Could you check a few things on this drawing? It's one solid part, dimensions in mm from its lowest x, y, z. A direction names the side the tool comes from. Coordinates: 2 decimals unless noted, no trailing zeros. Order: outer loops, then holes, each group sorted by start corner. A loop starts at its lowest first (then second) coordinate and runs counter-clockwise, first axis right, second up.
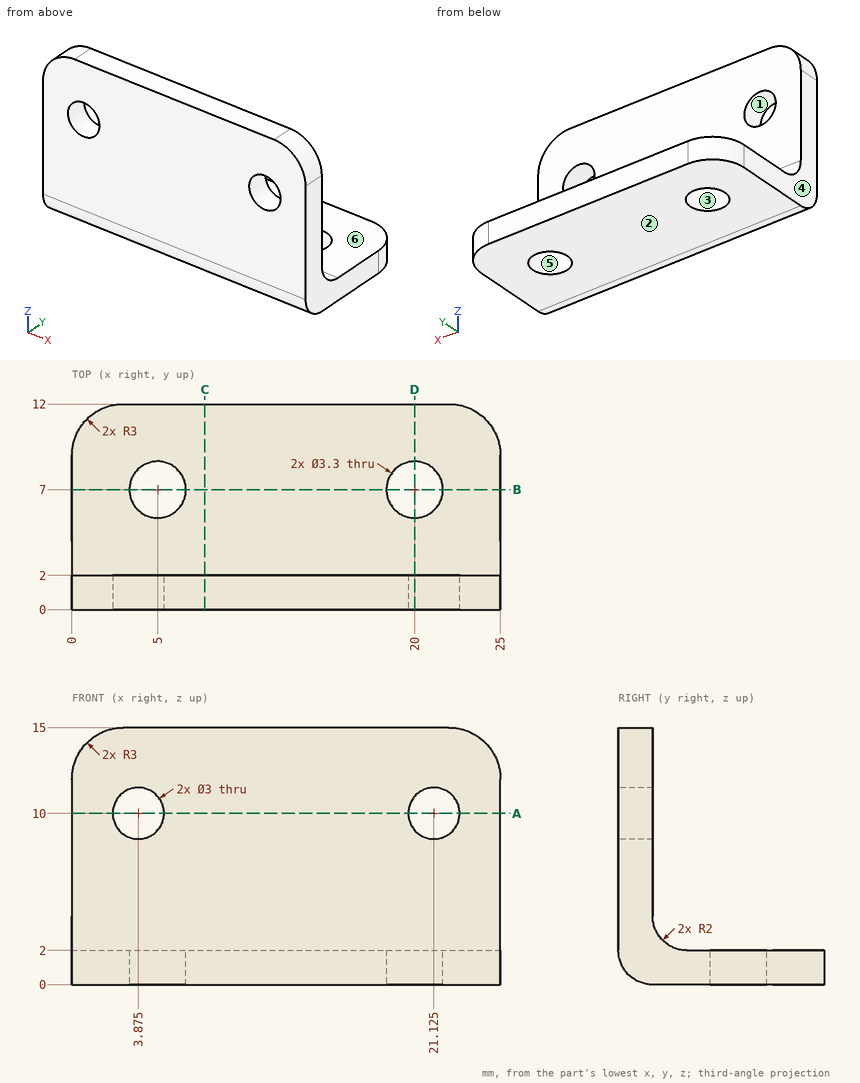
Item 1: Which directions (+Z, -Z, +X, -X, +Y, -Y) give clear straight access to the entire face, cutting with the end or side of a thin tool? Please do the marked faces 5 and 6.
Item 2: Suppose I cut it at D-D (x = 20). List the corners of the cut face in (y, z) for me.
Item 3: Suppose I cut it at C-C (x = 7.75). List the corners of the cut face in (y, z) for me.
Item 4: I need wall thicknesses on line 1 (X direction, y = 7, z = 1.35); line 2 (Y direction, x = 7.5, z = 9.75); line 3 (X direction, y = 1.75, z = 9.75). Which ranges of each line are inside material? Lowest first, please.
Item 5: For pin 1 Ø4 at (x, y) = (11.5, 8.5) entering from +Z; pin 2 Ø9 at (x, z) = (6.5, 7.5) entering from +Y, each with a flat end and sliding along its axis, tell me the tip position at first contact or that it passes through.
Item 6: Thinking about a two-plate mould opening in X: for the marked faces 1, 2, 3 and 4, which applies, +X half, -X half, draft (parallel to the pull), parting line (faces both ways), or undercut?
Item 7: Suppose I cut it at B-B (y = 7). List the corners of the cut face in (x, z) for me.
Item 8: Suppose I cut it at A-A (z = 10). List the corners of the cut face in (x, y) for me (3 decimals), and give its area (3 significant figures).
Geometry results:
1. face 5: +Z, -Z
1. face 6: +Z, +X, -X, +Y
2. outline: (0, 2) arc R2 ccw to (2, 0) - (5.35, 0) - (5.35, 2) - (4, 2) arc R2 cw to (2, 4) - (2, 9.01) - (0, 9.01) - close; (0, 10.99) - (2, 10.99) - (2, 15) - (0, 15) - close; (8.65, 0) - (12, 0) - (12, 2) - (8.65, 2) - close
3. outline: (0, 2) arc R2 ccw to (2, 0) - (12, 0) - (12, 2) - (4, 2) arc R2 cw to (2, 4) - (2, 15) - (0, 15) - close
4. line 1: x = 0 to 3.35, 6.65 to 18.35, 21.65 to 25
4. line 2: y = 0 to 2
4. line 3: x = 0 to 2.4, 5.35 to 19.65, 22.6 to 25
5. pin 1: stops at z = 2
5. pin 2: stops at y = 2.27
6. face 1: undercut
6. face 2: draft
6. face 3: undercut
6. face 4: -X half
7. outline: (0, 0) - (3.35, 0) - (3.35, 2) - (0, 2) - close; (6.65, 0) - (18.35, 0) - (18.35, 2) - (6.65, 2) - close; (21.65, 0) - (25, 0) - (25, 2) - (21.65, 2) - close
8. outline: (0, 0) - (2.375, 0) - (2.375, 2) - (0, 2) - close; (5.375, 0) - (19.625, 0) - (19.625, 2) - (5.375, 2) - close; (22.625, 0) - (25, 0) - (25, 2) - (22.625, 2) - close
8. area: 38.0 mm2
